Source: CAD feature listing. Evaluate the final solid. Frame: model axes, mm. A direction names the side the tool comes from. Give positions to 0.01 mm unless a question says otherwise; leave off trailing zeros. Order: outer loops, then holes, each group sorted by start corner. A loop starts at its lowest first (then second) coordinate and runs counter-clockwise, first axis right, second up. Notation, with made-up numbers: M -3.75,52.25 L 30.25,52.25 A12 cw 30.25,72.25 Z; hole C 17.25,48.25 d10. An arc over 180 degrees is marked long. Answer in a Markdown table with one row per item. Add a question column.
(1) Mould query, pull axis Z, two halves, no side actions, for faces 1 (the face through (-17, 0, 29)), 2 (the face through (28, -2, 10)), 3 (the face through (10, 3, 0)), 4 (the face through (-22.989, 19.233, 4.93)). Classes: pulls with the +Z half, pulls with the -Z half, needs draft (parallel to the pull), parting line crosses it, or undercut.
(2) Section query D-D, the plane z = 35.5. Return loops of the section in (x, y).
(3) Section query A-A, the plane y = 0. Return loops of the section in (x, z).
(4) Section query C-C, the plane y = -7.5. Return loops of the section in (x, z).
(5) Pin query (flat end, axial travel): P1, Ø19, axis at x = -35, y = 0, coming from the +Z side; P2, Ø8, axis at x = 33.5, z = 14.5, coming from the -Y side; P3, Ø6, axis at x = -5, z = 25, coming from the -Y side; P4, Ø1.5, axis at x = -23, z = 33, coming from the -Y side. Return the tip coordinate at first contact, or that it passes through.
(6) Section query B-B, the plane x = 0. Return loops of the section in (y, z), plus the area to 3 significant figures.
(7) Set-up query: faces 5 (the face through (50, 0, 5)), 6 (the face through (-14.985, 0.66, 35.042)). Return all of +Z, -Z, +X, -X, +Y, -Y with unobstructed straight access to the full face (end or side cutting, diameter ignored); none if empty.
(8) Material intervals for line 1 along Y through (x, z) = (0, 10); line 2 along Y through (x, z) = (0, 35.25); line 3 along X through (y, z) = (20, 13.5), sorted ascending.
from build123d import *

# Parameters (mm, degrees)
SKETCH1_R                                 = 6
BOSS_EXTRUDE1_DEPTH                       = 10
BOSS_EXTRUDE1_2_DEPTH                     = 10
SKETCH1_3_R                               = 25
BOSS_EXTRUDE2_DEPTH                       = 38
CBORE_FOR_M12_HEX_HEAD_SCREW1_D           = 20
CBORE_FOR_M12_HEX_HEAD_SCREW1_CBORE_D     = 30
CBORE_FOR_M12_HEX_HEAD_SCREW1_CBORE_DEPTH = 6
SKETCH6_R                                 = 3
CUT_EXTRUDE1_DEPTH                        = 38


with BuildPart() as part:
    # Sketch1 → Boss-Extrude1 (new body)
    with BuildSketch(Plane.XY):
        with BuildLine():
            Line((-7.142857143, 23.957871187), (-39.285714286, 14.374722712))
            ThreePointArc((-39.285714286, 14.374722712), (-50, 0), (-39.285714286, -14.374722712))
            Line((-39.285714286, -14.374722712), (-7.142857143, -23.957871187))
            ThreePointArc((-7.142857143, -23.957871187), (-25, 0), (-7.142857143, 23.957871187))
        make_face()
        with Locations((-35, 0)):
            Circle(SKETCH1_R, mode=Mode.SUBTRACT)
    extrude(amount=BOSS_EXTRUDE1_DEPTH)



with BuildPart() as body_2:
    # Sketch1 → Boss-Extrude1 2 (new body)
    with BuildSketch(Plane.XY):
        with BuildLine():
            Line((39.285714286, 14.374722712), (7.142857143, 23.957871187))
            ThreePointArc((7.142857143, 23.957871187), (20.044593143, 14.940357617), (25, 0))
            ThreePointArc((25, 0), (20.044593143, -14.940357617), (7.142857143, -23.957871187))
            Line((7.142857143, -23.957871187), (39.285714286, -14.374722712))
            ThreePointArc((39.285714286, -14.374722712), (50, 0), (39.285714286, 14.374722712))
        make_face()
        with Locations((35, 0)):
            Circle(SKETCH1_R, mode=Mode.SUBTRACT)
    extrude(amount=BOSS_EXTRUDE1_2_DEPTH)


with BuildPart() as part_1:
    add(part.part)

    add(body_2.part)  # Boss-Extrude2 merges body 2
    # Sketch1_3 → Boss-Extrude2 (add)
    with BuildSketch(Plane.XY):
        with Locations(Location((0, 0, 0), (0, 0, 106.601549599))):
            Circle(SKETCH1_3_R)
    extrude(amount=BOSS_EXTRUDE2_DEPTH)

    # CBORE for M12 Hex Head Screw1 (through all)
    with Locations(Plane.XY.offset(38)):
        with Locations((0, 0)):
            CounterBoreHole(CBORE_FOR_M12_HEX_HEAD_SCREW1_D / 2, CBORE_FOR_M12_HEX_HEAD_SCREW1_CBORE_D / 2, CBORE_FOR_M12_HEX_HEAD_SCREW1_CBORE_DEPTH)

    # Sketch6 → Cut-Extrude1 (cut)
    with BuildSketch(Plane(origin=(0, 0, 0), x_dir=(0, 0, -1), z_dir=(1, 0, 0))):
        with Locations((-26, 0)):
            Circle(SKETCH6_R)
    extrude(amount=-CUT_EXTRUDE1_DEPTH, mode=Mode.SUBTRACT)


solid = part_1.part
Values follow:
| question | item | result |
|---|---|---|
| 1 | face 1 | undercut |
| 1 | face 2 | pulls with the +Z half |
| 1 | face 3 | pulls with the -Z half |
| 1 | face 4 | needs draft |
| 2 | outline | C 0,0 d50; hole C 0,0 d30 |
| 3 | outline | M -50,0 L -41,0 L -41,10 L -50,10 Z; M -29,0 L -10,0 L -10,23 L -25,23 L -25,10 L -29,10 Z; M -25,29 L -10,29 L -10,32 L -15,32 L -15,38 L -25,38 Z; M 10,0 L 29,0 L 29,10 L 25,10 L 25,38 L 15,38 L 15,32 L 10,32 Z; M 41,0 L 50,0 L 50,10 L 41,10 Z |
| 4 | outline | M -47.99,0 L -6.61,0 L -6.61,32 L -12.99,32 L -12.99,38 L -23.85,38 L -23.85,10 L -47.99,10 Z; M 6.61,0 L 47.99,0 L 47.99,10 L 23.85,10 L 23.85,38 L 12.99,38 L 12.99,32 L 6.61,32 Z |
| 5 | P1 | stops at z = 10 |
| 5 | P2 | passes through |
| 5 | P3 | stops at y = -24.92 |
| 5 | P4 | stops at y = -11.4 |
| 6 | outline | M -25,0 L -10,0 L -10,32 L -15,32 L -15,38 L -25,38 Z; M 10,0 L 25,0 L 25,38 L 15,38 L 15,32 L 10,32 Z |
| 6 | area | 1,080 mm² |
| 7 | face 5 | +Z, -Z, +X |
| 7 | face 6 | +Z |
| 8 | line 1 | y = -25 to -10, 10 to 25 |
| 8 | line 2 | y = -25 to -15, 15 to 25 |
| 8 | line 3 | x = -15 to 15 |
